from build123d import *

# Parameters (mm, degrees)
CROQUIS1_R              = 1.5
CROQUIS1_W              = 15
CROQUIS1_H              = 2
SALIENTE_EXTRUIR1_DEPTH = 3.5
CORTAR_EXTRUIR1_START   = -3.5
CORTAR_EXTRUIR1_DEPTH   = 3.5
REDONDEO1_R             = 4
REDONDEO3_R             = 1


with BuildPart() as part:
    # Croquis1 → Saliente-Extruir1 (new, symmetric)
    with BuildSketch(Plane(origin=(0, 0, 0), x_dir=(0, 0, -1), z_dir=(1, 0, 0))):
        with BuildLine():
            Line((4.197209499, 4), (-18.186825032, 14.437846722))
            ThreePointArc((-18.186825032, 14.437846722), (-22.173603178, 12.986778146), (-20.722534603, 9))
            Line((-20.722534603, 9), (-10, 4))
            Line((-10, 4), (-10, -4))
            Line((-10, -4), (10, -4))
            Line((10, -4), (10, 4))
            Line((10, 4), (4.197209499, 4))
        make_face()
        with Locations((-19.454679817, 11.718923361)):
            Circle(CROQUIS1_R, mode=Mode.SUBTRACT)
        with Locations((0, 1)):
            Rectangle(CROQUIS1_W, CROQUIS1_H, mode=Mode.SUBTRACT)
    extrude(amount=SALIENTE_EXTRUIR1_DEPTH, both=True)

    # Croquis2 → Cortar-Extruir1 (cut)
    with BuildSketch(Plane.ZY.offset(3.5).offset(CORTAR_EXTRUIR1_START)):
        with BuildLine():
            Line((-4.197209499, 4), (10, 4))
            Line((10, 4), (20.722534603, 9))
            ThreePointArc((20.722534603, 9), (22.173603178, 12.986778146), (18.186825032, 14.437846722))
            Line((18.186825032, 14.437846722), (-4.197209499, 4))
        make_face()
    extrude(amount=CORTAR_EXTRUIR1_DEPTH, mode=Mode.SUBTRACT)

    # Redondeo1
    # the kernel refuses this fillet: 4 mm, written as the material it adds along each edge
    with BuildSketch(Plane(origin=(0, 4, -14.118776915), x_dir=(-1, 0, 0), z_dir=(0, 0, 1))) as redondeo1_piece_1_section:
        with BuildLine():
            CenterArc((4, -3.968626967), REDONDEO1_R, 97.180755781, 82.819244219)
            Line((0, -3.968626967), (0, 0))
            Line((0, 0), (3.5, 0))
        make_face()
    redondeo1_piece_1 = extrude(amount=24.118776915, mode=Mode.PRIVATE)
    redondeo1_piece_1 = split(redondeo1_piece_1, bisect_by=Plane(origin=(0, 0.199819207, -12.346723509), z_dir=(0, -0.9063077870366529, 0.42261826174069317)), keep=Keep.TOP, mode=Mode.PRIVATE)
    redondeo1_piece_1 = split(redondeo1_piece_1, bisect_by=Plane(origin=(0, -5.238027515, -9.811013939), z_dir=(0, 0.9063077870366527, -0.4226182617406936)), keep=Keep.TOP, mode=Mode.PRIVATE)
    add(redondeo1_piece_1)
    with BuildSketch(Plane(origin=(0, 4, -14.118776915), x_dir=(-1, 0, 0), z_dir=(0, 0, 1))) as redondeo1_piece_2_section:
        with BuildLine():
            CenterArc((4, -3.968626967), REDONDEO1_R, 97.180755781, 82.819244219)
            Line((0, -3.968626967), (0, 0))
            Line((0, 0), (3.5, 0))
        make_face()
    redondeo1_piece_2 = extrude(amount=34.040344332, mode=Mode.PRIVATE)
    redondeo1_piece_2 = split(redondeo1_piece_2, bisect_by=Plane(origin=(0, 4, 10), z_dir=(0, 0, 1)), keep=Keep.TOP, mode=Mode.PRIVATE)
    redondeo1_piece_2 = split(redondeo1_piece_2, bisect_by=Plane(origin=(0, -5.238027515, -9.811013939), z_dir=(0, 0.9063077870366527, -0.4226182617406936)), keep=Keep.TOP, mode=Mode.PRIVATE)
    add(redondeo1_piece_2)
    # the kernel refuses this fillet: 4 mm, written as the material it adds along each edge
    with BuildSketch(Plane(origin=(-3.5, 4, -4.197209499), x_dir=(0, 0, -1), z_dir=(1, 0, 0))) as redondeo1_2_piece_1_section:
        with BuildLine():
            CenterArc((REDONDEO1_R * 0.221694662643, REDONDEO1_R), REDONDEO1_R, 245, 25)
            Line((-REDONDEO1_R * 0.200923599098, REDONDEO1_R * 0.0936922129633), (0, 0))
            Line((0, 0), (REDONDEO1_R * 0.221694662643, 0))
        make_face()
    redondeo1_2_piece_1 = extrude(amount=7, mode=Mode.PRIVATE)
    redondeo1_2_piece_1 = redondeo1_2_piece_1 - Plane(origin=(-4, 7.968626967, -4.197209499), x_dir=(0.12499999999999983, -0.9921567416492215, 0), z_dir=(0, 0, -1)) * Cylinder(4, 18, mode=Mode.PRIVATE)
    add(redondeo1_2_piece_1)

    # Redondeo3
    redondeo3_edges = [part.edges().sort_by_distance(p)[0] for p in [
        (0, -4, -10),
        (0, -4, 10),
        (0, 4, -10),
    ]]
    fillet(redondeo3_edges, radius=REDONDEO3_R)


solid = part.part
Design review of the part built by this model. Coordinates are the model's own, in mm. A direction names the side the tool comes from. Coordinates: 2 decimals unless noted, no trailing zeros. Order: outer loops, then holes, each group sorted by start corner. A loop starts at its lowest first (then second) coordinate and runs counter-clockwise, first axis right, second up.
Item 1: The part is to be moulded in two halves that separate along Y. For faces 1 (the flat face through (0, 0, 0)), 2 (the cylindrical face through (-0.049, -3.699, -9.715)), 3 (the flat face through (0, 0, -10)), 4 (the flat face through (0, 1, 7.5)), say which applies: pulls with the +Y half, pulls with the -Y half, needs draft (parallel to the pull), parting line crosses it, or undercut.
Item 2: Take a section at B-B, the plane x = 2.75. Write out the cut boundary in (y, z), then the cut area to 3 significant figures.
Item 3: For line 1 (Z direction, x = -2.5, y = 1.75); line 2 (Y direction, x = 0.75, z = -5); line 3 (Z direction, x = -3, y = -1.25), list the stretches that pass through material, from the lowest coordinate up.
Item 4: For faces 5 (the flat face through (0, 0, 10)), 6 (the flat face through (0, 2, 0)), 7 (the flat face through (0, 11, 15)), 8 (the flat face through (0, 4, -7)), list the 3-axis set-ups (+Z, -Z, +X, -X, +Y, -Y) from which the entire face can be reached by the end or side of a thin tool; tool diameter is ignored.
Item 5: For pin 1 Ø3.5 at (y, z) = (11.72, 19.45) entering from +X; pin 2 Ø1 at (x, y) = (0, 1.5) entering from +Z; pin 3 Ø1 at (x, z) = (0, 10.5) entering from +Y; pin 4 Ø1.5 at (x, z) = (2, 13.5) entering from +Y, all flat-tipped, find the tip position at first contact; note any pin that passes through.
Item 6: Take a section at A-A, the plane y = 0.5. Write out the cut boundary in (x, z).
Item 7: Take a section at C-C, the plane z = 20. Write out the cut boundary in (x, y), then the cut area to 3 significant figures.
Item 8: Take a section at D-D, the plane x = -0.5. Write out the cut boundary in (y, z), then the cut area to 3 significant figures.
The answers:
1. face 1: undercut
1. face 2: pulls with the -Y half
1. face 3: needs draft
1. face 4: undercut
2. outline: (-4, -9) arc R1 ccw to (-3, -10) - (3, -10) arc R1 ccw to (4, -9) - (4, -5.08) arc R4 cw to (4.37, -3.39) - (14.44, 18.19) arc R3 ccw to (9, 20.72) - (4, 10) - (-3, 10) arc R1 ccw to (-4, 9) - close; hole (0, -7.5) - (2, -7.5) - (2, 7.5) - (0, 7.5) - close; hole circle Ø3 at (11.72, 19.45)
2. area: 246 mm2
3. line 1: z = -10 to -7.5, 7.5 to 10
3. line 2: y = -4 to 0, 2 to 4
3. line 3: z = -10 to 10
4. face 5: +Z, +X, -X, -Y
4. face 6: +X, -X
4. face 7: +Z, -Z, -X, +Y
4. face 8: -Z, +X, -X, +Y
5. pin 1: stops at x = 3.5
5. pin 2: stops at z = 10
5. pin 3: stops at y = 11.09
5. pin 4: stops at y = 12.6
6. outline: (-3.5, -10) - (3.5, -10) - (3.5, -7.5) - (-3.5, -7.5) - close; (-3.5, 7.5) - (3.5, 7.5) - (3.5, 10) - (-3.5, 10) - close
7. outline: (0, 8.66) - (3.5, 8.66) - (3.5, 10.32) - (0, 10.32) - close; (0, 13.12) - (3.5, 13.12) - (3.5, 14.67) - (0, 14.67) - close
7. area: 11.2 mm2
8. outline: (-4, -9) arc R1 ccw to (-3, -10) - (3, -10) arc R1 ccw to (4, -9) - (4, -5.08) arc R4 cw to (4.37, -3.39) - (6.03, 0.16) - (6.03, 14.36) - (4, 10) - (-3, 10) arc R1 ccw to (-4, 9) - close; hole (0, -7.5) - (2, -7.5) - (2, 7.5) - (0, 7.5) - close
8. area: 158 mm2
